Geometry: final body of the model. Coordinates: model frame, mm. A direction names the side the tool comes from. Give positions to 0.01 mm unless a question says otherwise; leave off trailing zeros. Order: outer loops, then holes, each group sorted by start corner. A loop starts at its lowest first (then second) coordinate and runs counter-clockwise, first axis right, second up. Notation, with made-up numbers: (66.5, 8) -> (96.5, 8) arc R24 cw to (96.5, 34) -> close; hole circle Ø3 at (9, 67). An arc over 180 degrees is marked (long way). One line per question, with ' | ' between items.
from build123d import *

# Parameters (mm, degrees)
F1_DEPTH = 25.4
F2_R     = 3.5687
F3_DEPTH = 7.1374
F4_DEPTH = 7.1374


# Not quite as in the source:
# - a feature names something its author has since deleted; it is built from what else it names


with BuildPart() as f1:
    # F0 (on Front) → F1 (new body)
    with BuildSketch(Plane.XZ):
        with BuildLine():
            Line((47.6553842176, 38.1), (-47.5946157824, 38.1))
            Line((-47.5946157824, 38.1), (-47.5946157824, 0))
            Line((-47.5946157824, 0), (-18.3505333031, 0))
            ThreePointArc((-18.3505333031, 0), (0, 18.3505333031), (18.3505333031, 0))
            Line((18.3505333031, 0), (47.6553842176, 0))
            Line((47.6553842176, 0), (47.6553842176, 38.1))
        make_face()
        with BuildLine():
            Line((-18.3505333031, 0), (-47.5946157824, 0))
            Line((-47.5946157824, 0), (-47.5946157824, -38.1))
            Line((-47.5946157824, -38.1), (47.6553842176, -38.1))
            Line((47.6553842176, -38.1), (47.6553842176, 0))
            Line((47.6553842176, 0), (18.3505333031, 0))
            ThreePointArc((18.3505333031, 0), (0, -18.3505333031), (-18.3505333031, 0))
        make_face()
    extrude(amount=F1_DEPTH)

    # F2 (on face) → F3 (cut)
    with BuildSketch(Plane.XY.offset(38.1)):
        with Locations((37.3155283745, -12.5269582962)):
            Circle(F2_R)
    extrude(amount=-F3_DEPTH, mode=Mode.SUBTRACT)

    # F2 (on face) → F4 (cut)
    with BuildSketch(Plane.XY.offset(38.1)):
        with Locations((-38.8844716255, -12.6503112141)):
            Circle(F2_R)
        with Locations((37.3155283745, -12.5269582962)):
            Circle(F2_R)
    extrude(amount=-F4_DEPTH, mode=Mode.SUBTRACT)


solid = f1.part
1) Contact query for flat-ended pins moving along their axis: pin 1 Ø3.5 at (x, y) = (36.5, -13) entering from +Z; pin 2 Ø22 at (x, z) = (0, 0) entering from -Y. Output: stop coordinate, or through.
Check result:
pin 1: stops at z = 30.96 | pin 2: passes through
2) Material intervals for probe 1 along X at (y, z) = (-14.75, 0); probe 2 along Z at (x, y) = (0, -5.25); probe 3 along Z at (x, y) = (-10, -22), sorted ascending. Write a range as from..to.
Check result:
probe 1: x = -47.59..-18.35, 18.35..47.66 | probe 2: z = -38.1..-18.35, 18.35..38.1 | probe 3: z = -38.1..-15.39, 15.39..38.1
3) Section A-A on z = 0. Return loops of the section in (x, y), plus the area to 3 significant figures.
Check result:
outline: (-47.59, -25.4) -> (-18.35, -25.4) -> (-18.35, 0) -> (-47.59, 0) -> close; (18.35, -25.4) -> (47.66, -25.4) -> (47.66, 0) -> (18.35, 0) -> close | area: 1,490 mm^2
4) Set-up query: faces 4 (the flat face through (-39, -13, 30.963)), 5 (the flat face through (-47.595, -13, 1)). Return all of +Z, -Z, +X, -X, +Y, -Y with unobstructed straight access to the full face (end or side cutting, diameter ignored); none if empty.
Check result:
face 4: +Z | face 5: +Z, -Z, -X, +Y, -Y
5) Pull-direction query (Z, two-part tool) for faces 1 (the cylindrical face through (-3.978, -12.522, 17.914)), 2 (the flat face through (-1, -13, -38.1)), 3 (the cylindrical face through (40.612, -13.894, 34.581)); classes: +Z half, -Z half, draft (parallel to the pull), parting line (faces both ways), or undercut.
Check result:
face 1: undercut | face 2: -Z half | face 3: draft
6) Section B-B on x = 0. Return loops of the section in (y, z), plus the area to 3 significant figures.
Check result:
outline: (-25.4, -38.1) -> (0, -38.1) -> (0, -18.35) -> (-25.4, -18.35) -> close; (-25.4, 18.35) -> (0, 18.35) -> (0, 38.1) -> (-25.4, 38.1) -> close | area: 1,000 mm^2
7) Section C-C on y = -19.75. Return loops of the section in (x, z).
Check result:
outline: (-47.59, -38.1) -> (47.66, -38.1) -> (47.66, 38.1) -> (-47.59, 38.1) -> close; hole circle Ø36.7 at (0, 0)
8) Section D-D on x = -37. Return loops of the section in (y, z), plus the area to 3 significant figures.
Check result:
outline: (-25.4, -38.1) -> (0, -38.1) -> (0, 38.1) -> (-9.62, 38.1) -> (-9.62, 30.96) -> (-15.68, 30.96) -> (-15.68, 38.1) -> (-25.4, 38.1) -> close | area: 1,890 mm^2
